Can you work these out from the model? Positions are in its coordinate system, mm. Face numbers are marked on the shaded views. Round coordinates to 2 decimals unless told otherwise and drop trailing zeros. Loops run counter-clockwise (first coordinate to the right, second up) from the corner with the lowest first, then second, coordinate; pieces in that order, holes last. Notation, with made-up numbers: M 76,80 L 132,80 A9 ccw 132,85 Z; hole C 55,36.5 d9. An arc over 180 degrees is marked long. Return JSON: item names as keys, results as strings.
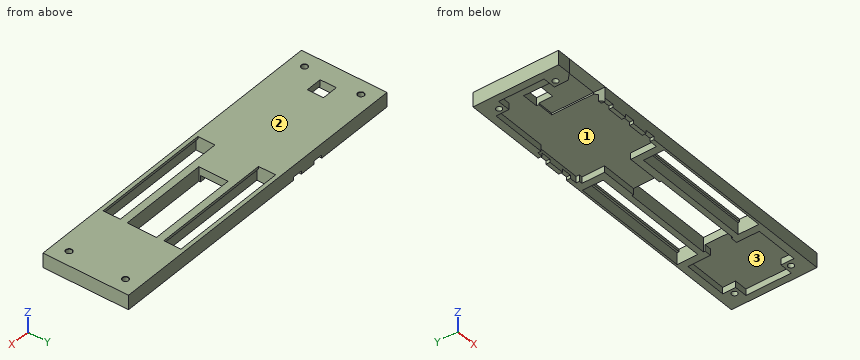
```python
from build123d import *

# Parameters (mm, degrees)
SKETCH_1_W                   = 101
SKETCH_1_H                   = 26.5
EXTRUDE_1_DEPTH              = 2.5
SKETCH_10_W                  = 37
SKETCH_10_H                  = 7
CUT_EXTRUDE_1_DEPTH          = 2.5
EXTRUDE_2_DEPTH              = 2
HOLE_WIZARD_M6_4_D           = 1.8
HOLE_WIZARD_M6_4_CSINK_D     = 2
HOLE_WIZARD_M6_4_CSINK_ANGLE = 90
EXTRUDE_START                = 2
SKETCH_17_W                  = 4
SKETCH_17_H                  = 4
SKETCH_17_R                  = 0.9
EXTRUDE_3_DEPTH              = 2
SKETCH_18_W                  = 42.1
SKETCH_18_H                  = 9.1
CUT_EXTRUDE_2_DEPTH          = 1
CUT_EXTRUDE_3_REACH          = 106.477
SKETCH_20_W                  = 28
SKETCH_20_H                  = 9.1
SKETCH_22_W                  = 0.8
SKETCH_22_H                  = 0.5
EXTRUDE_4_DEPTH              = 37
EXTRUDE_5_DEPTH              = 1
SKETCH_24_W                  = 10
SKETCH_24_H                  = 2.5
SKETCH_24_W_2                = 3
SKETCH_24_H_2                = 1
CUT_EXTRUDE_4_DEPTH          = 15
CHAMFER_1_SIZE               = 2
CUT_EXTRUDE_5_REACH          = 106.449
SKETCH_25_W                  = 3
SKETCH_25_H                  = 1
SKETCH_27_W                  = 5
SKETCH_27_H                  = 5
CUT_EXTRUDE_6_DEPTH          = 9
SKETCH_28_W                  = 15
SKETCH_28_H                  = 1
SKETCH_28_W_2                = 23.55
CUT_EXTRUDE_7_DEPTH          = 2


with BuildPart() as part:
    # 草图1 → 凸台-拉伸1 (new body)
    with BuildSketch(Plane.XY):
        with Locations((50.5, 13.25)):
            Rectangle(SKETCH_1_W, SKETCH_1_H)
    extrude(amount=EXTRUDE_1_DEPTH)

    # 草图10 → 切除-拉伸1 (cut)
    with BuildSketch(Plane.XY.offset(2.5)):
        with Locations((60.5, 23)):
            Rectangle(SKETCH_10_W, SKETCH_10_H)
        with Locations((60.5, 3.5)):
            Rectangle(SKETCH_10_W, SKETCH_10_H)
    extrude(amount=-CUT_EXTRUDE_1_DEPTH, mode=Mode.SUBTRACT)

    # 草图11 → 凸台-拉伸2 (add)
    with BuildSketch(Plane(origin=(0, 0, 0), x_dir=(-1, 0, 0), z_dir=(0, 0, -1))):
        Polygon((-42, 26.5), (-42, 19.5), (-79, 19.5), (-79, 26.5), (-101, 26.5), (-101, 0), (-79, 0), (-79, 7), (-42, 7), (-42, 0), (0, 0), (0, 26.5), align=None)
        Polygon((-39.8, 24.3), (-39.8, 17.3), (-81.2, 17.3), (-81.2, 24.3), (-98.8, 24.3), (-98.8, 2.2), (-81.2, 2.2), (-81.2, 9.2), (-39.8, 9.2), (-39.8, 2.2), (-2.2, 2.2), (-2.2, 24.3), align=None, mode=Mode.SUBTRACT)
    extrude(amount=EXTRUDE_2_DEPTH)

    # M6 开槽半沉头螺钉的锥形沉头孔4 (through all)
    with Locations(Plane(origin=(0, 0, 2.5), x_dir=(-1, 0, 0), z_dir=(0, 0, 1))):
        with Locations((-4.5, -4.5), (-96.5, -22), (-96.5, -4.5), (-4.5, -22)):
            CounterSinkHole(HOLE_WIZARD_M6_4_D / 2, HOLE_WIZARD_M6_4_CSINK_D / 2, counter_sink_angle=HOLE_WIZARD_M6_4_CSINK_ANGLE)

    # 草图17 → 凸台-拉伸3 (add)
    # profile 1 of 4: a face of its own
    with BuildSketch(Plane(origin=(0, 0, 0), x_dir=(-1, 0, 0), z_dir=(0, 0, -1)).offset(EXTRUDE_START)):
        with Locations((-96.8, 22.3)):
            Rectangle(SKETCH_17_W, SKETCH_17_H)
        with Locations(Location((-96.5, 22, 0), (0, 0, 180))):
            Circle(SKETCH_17_R, mode=Mode.SUBTRACT)
    # profile 2 of 4: a face of its own
    with BuildSketch(Plane(origin=(0, 0, 0), x_dir=(-1, 0, 0), z_dir=(0, 0, -1)).offset(EXTRUDE_START)):
        with Locations((-96.8, 4.2)):
            Rectangle(SKETCH_17_W, SKETCH_17_H)
        with Locations(Location((-96.5, 4.5, 0), (0, 0, 180))):
            Circle(SKETCH_17_R, mode=Mode.SUBTRACT)
    # profile 3 of 4: a face of its own
    with BuildSketch(Plane(origin=(0, 0, 0), x_dir=(-1, 0, 0), z_dir=(0, 0, -1)).offset(EXTRUDE_START)):
        with Locations((-4.2, 22.3)):
            Rectangle(SKETCH_17_W, SKETCH_17_H)
        with Locations(Location((-4.5, 22, 0), (0, 0, 180))):
            Circle(SKETCH_17_R, mode=Mode.SUBTRACT)
    # profile 4 of 4: a face of its own
    with BuildSketch(Plane(origin=(0, 0, 0), x_dir=(-1, 0, 0), z_dir=(0, 0, -1)).offset(EXTRUDE_START)):
        with Locations((-4.2, 4.2)):
            Rectangle(SKETCH_17_W, SKETCH_17_H)
        with Locations(Location((-4.5, 4.5, 0), (0, 0, 180))):
            Circle(SKETCH_17_R, mode=Mode.SUBTRACT)
    extrude(amount=-EXTRUDE_3_DEPTH)

    # 草图18 → 切除-拉伸2 (cut)
    with BuildSketch(Plane.XY.offset(2.5)):
        Polygon((37, 8.7), (37, 17.8), (37, 19.5), (32, 19.5), (32, 7), (37, 7), align=None)
        with Locations((58.05, 13.25)):
            Rectangle(SKETCH_18_W, SKETCH_18_H)
        Polygon((79.1, 19.5), (79.1, 17.8), (79.1, 8.7), (79.1, 7), (84.1, 7), (84.1, 19.5), align=None)
    extrude(amount=-CUT_EXTRUDE_2_DEPTH, mode=Mode.SUBTRACT)

    # 草图20 → 切除-拉伸3 (cut, up to next)
    with BuildSketch(Plane.XY.offset(1.5), mode=Mode.PRIVATE) as cut_extrude_3_sk1:
        with Locations((65.1, 13.25)):
            Rectangle(SKETCH_20_W, SKETCH_20_H)
    cut_extrude_3_tool1 = extrude(cut_extrude_3_sk1.sketch, amount=-CUT_EXTRUDE_3_REACH, mode=Mode.PRIVATE) & part.part
    add(cut_extrude_3_tool1.solids().sort_by_distance((65.1, 13.25, 1.5))[0], mode=Mode.SUBTRACT)

    # 草图22 → 凸台-拉伸4 (add)
    with BuildSketch(Plane.ZY.offset(-79)):
        Polygon((-2, 26.5), (2.5, 26.5), (2.5, 25.35398434), (2.5, 25.3), (1.7, 25.3), (1.7, 25.9), (-2, 25.9), align=None)
        with Locations((2.1, 19.75)):
            Rectangle(SKETCH_22_W, SKETCH_22_H)
        with Locations((2.1, 6.75)):
            Rectangle(SKETCH_22_W, SKETCH_22_H)
        Polygon((-2, 0.6), (-2, 0), (2.5, 0), (2.5, 1.14601566), (2.5, 1.2), (1.7, 1.2), (1.7, 0.6), align=None)
    extrude(amount=EXTRUDE_4_DEPTH)

    # 草图23 → 凸台-拉伸5 (add)
    with BuildSketch(Plane.XY.offset(1.5)):
        Polygon((84.1, 7), (84.1, 19.5), (79.1, 19.5), (79.1, 17.8), (79.1, 8.7), (79.1, 7), align=None)
        Polygon((51.1, 8.7), (51.1, 17.8), (37, 17.8), (37, 19.5), (32, 19.5), (32, 7), (37, 7), (37, 8.7), align=None)
    extrude(amount=EXTRUDE_5_DEPTH)

    # 草图24 → 切除-拉伸4 (cut)
    with BuildSketch(Plane.XZ):
        with Locations((11.25, -0.75)):
            Rectangle(SKETCH_24_W, SKETCH_24_H)
        with Locations((19.75, -1.5)):
            Rectangle(SKETCH_24_W_2, SKETCH_24_H_2)
        with Locations((27.75, -1.5)):
            Rectangle(SKETCH_24_W_2, SKETCH_24_H_2)
        with Locations((35.75, -1.5)):
            Rectangle(SKETCH_24_W_2, SKETCH_24_H_2)
    extrude(amount=-CUT_EXTRUDE_4_DEPTH, mode=Mode.SUBTRACT)

    # 倒角1
    chamfer_1_edges = [part.edges().sort_by_distance(p)[0] for p in [
        (6.25, 0, -0.75),
        (16.25, 0, -0.75),
        (11.25, 0, 0.5),
    ]]
    chamfer(chamfer_1_edges, length=CHAMFER_1_SIZE - 0.0001)  # a hair under: the kernel refuses the full size

    # 草图25 → 切除-拉伸5 (cut, up to next)
    with BuildSketch(Plane(origin=(0, 26.5, 0), x_dir=(1, 0, 0), z_dir=(0, 1, 0)), mode=Mode.PRIVATE) as cut_extrude_5_sk1:
        with Locations((27, 1.5)):
            Rectangle(SKETCH_25_W, SKETCH_25_H)
    cut_extrude_5_tool1 = extrude(cut_extrude_5_sk1.sketch, amount=-CUT_EXTRUDE_5_REACH, mode=Mode.PRIVATE) & part.part
    # 草图25 → 切除-拉伸5 (cut, up to next)
    with BuildSketch(Plane(origin=(0, 26.5, 0), x_dir=(1, 0, 0), z_dir=(0, 1, 0)), mode=Mode.PRIVATE) as cut_extrude_5_sk2:
        with Locations((35, 1.5)):
            Rectangle(SKETCH_25_W, SKETCH_25_H)
    cut_extrude_5_tool2 = extrude(cut_extrude_5_sk2.sketch, amount=-CUT_EXTRUDE_5_REACH, mode=Mode.PRIVATE) & part.part
    add(cut_extrude_5_tool1.solids().sort_by_distance((27, 26.5, -1.5))[0], mode=Mode.SUBTRACT)
    add(cut_extrude_5_tool2.solids().sort_by_distance((35, 26.5, -1.5))[0], mode=Mode.SUBTRACT)

    # 草图27 → 切除-拉伸6 (cut)
    with BuildSketch(Plane(origin=(0, 0, 0), x_dir=(-1, 0, 0), z_dir=(0, 0, -1))):
        with Locations((-8.7, 13.2)):
            Rectangle(SKETCH_27_W, SKETCH_27_H)
    extrude(amount=-CUT_EXTRUDE_6_DEPTH, mode=Mode.SUBTRACT)

    # 草图28 → 切除-拉伸7 (cut)
    with BuildSketch(Plane(origin=(0, 0, -2), x_dir=(-1, 0, 0), z_dir=(0, 0, -1))):
        with Locations((-31.3, 24.8)):
            Rectangle(SKETCH_28_W, SKETCH_28_H)
        with Locations((-28.025, 1.7)):
            Rectangle(SKETCH_28_W_2, SKETCH_28_H)
    extrude(amount=-CUT_EXTRUDE_7_DEPTH, mode=Mode.SUBTRACT)


solid = part.part
```
Q1. I'm going to push flat-ended pins straight in: pin 1 Ø1 at (x, y) = (20, 0.5) entering from -Z; pin 2 Ø1.5 at (x, y) = (86, 16.5) entering from -Z; pin 3 Ø1.3 at (y, z) = (24, 0) entering from -X; pin 4 Ø0.7 at (x, y) = (67.5, 25.5) entering from -Z. Where does each tip first touch, or does it pass through?
Results:
{"pin 1": "stops at z = -1", "pin 2": "stops at z = 0", "pin 3": "stops at x = 0", "pin 4": "stops at z = 1.7"}
Q2. Suppose I cut it at A-A, the plane x = 96.5. Please give me the cut outline in (y, z), plus the area to 3 significant figures.
Results:
{"outline": "M 0,-2 L 3.6,-2 L 3.6,2.4 L 3.5,2.5 L 0,2.5 Z; M 5.4,-2 L 6.2,-2 L 6.2,0 L 20.3,0 L 20.3,-2 L 21.1,-2 L 21.1,2.4 L 21,2.5 L 5.5,2.5 L 5.4,2.4 Z; M 22.9,-2 L 26.5,-2 L 26.5,2.5 L 23,2.5 L 22.9,2.4 Z", "area": "74.8 mm2"}
Q3. Suppose I cut it at C-C, the plane y = 22. Please give me the cut outline in (x, z).
Results:
{"outline": "M 0,-2 L 3.6,-2 L 3.6,2.4 L 3.5,2.5 L 0,2.5 Z; M 5.4,-2 L 6.2,-2 L 6.2,0 L 39.8,0 L 39.8,-2 L 42,-2 L 42,2.5 L 5.5,2.5 L 5.4,2.4 Z; M 79,-2 L 81.2,-2 L 81.2,0 L 94.8,0 L 94.8,-2 L 95.6,-2 L 95.6,2.4 L 95.5,2.5 L 79,2.5 Z; M 97.4,-2 L 101,-2 L 101,2.5 L 97.5,2.5 L 97.4,2.4 Z"}
Q4. Thinking about a two-plate mould opening in X: for the marked faces 1, 2 and 3, which applies, pulls with the +X half, pulls with the -X half, needs draft (parallel to the pull), parting line crosses it, or undercut?
Results:
{"face 1": "undercut", "face 2": "needs draft", "face 3": "undercut"}
Q5. If I drill on line 1 along X through (y, z) = (22, 0.05); line 2 along Y through (x, z) = (44, 0.2); line 3 along X through (y, z) = (3, -0.4), over which ranges is the centre line in solid material (lowest first)?
Results:
{"line 1": "x = 0 to 3.6, 5.4 to 42, 79 to 95.6, 97.4 to 101", "line 2": "y = 0 to 0.6, 7 to 19.5, 25.9 to 26.5", "line 3": "x = 0 to 6.2, 39.8 to 42, 79 to 81.2, 94.8 to 101"}
Q6. Suppose I cut it at D-D, the plane x = 57. Please give me the cut outline in (y, z), plus the area to 3 significant figures.
Results:
{"outline": "M 0,-2 L 0.6,-2 L 0.6,1.7 L 1.2,1.7 L 1.2,2.5 L 0,2.5 Z; M 6.5,1.7 L 7,1.7 L 7,-2 L 8.7,-2 L 8.7,2.5 L 6.5,2.5 Z; M 17.8,-2 L 19.5,-2 L 19.5,1.7 L 20,1.7 L 20,2.5 L 17.8,2.5 Z; M 25.3,1.7 L 25.9,1.7 L 25.9,-2 L 26.5,-2 L 26.5,2.5 L 25.3,2.5 Z", "area": "22.5 mm2"}
Q7. Suppose I cut it at B-B, the plane y = 12.75. Please give me the cut outline in (x, z), plus the area to 3 significant figures.
Results:
{"outline": "M 0,-2 L 2.2,-2 L 2.2,0 L 6.2,0 L 6.2,2.5 L 0,2.5 Z; M 11.2,0.5 L 16.25,0.5 L 16.25,0 L 51.1,0 L 51.1,2.5 L 11.2,2.5 Z; M 79.1,0 L 98.8,0 L 98.8,-2 L 101,-2 L 101,2.5 L 79.1,2.5 Z", "area": "176 mm2"}
